Could you check a few things on this model? Use its own coordinates, in mm. A direction names the side the tool comes from. Give positions to 0.01 mm unless a question says otherwise; leave off trailing zeros. Order: outer loops, then holes, each group sorted by start corner. A loop starts at its lowest first (then second) coordinate and runs counter-clockwise, first axis right, second up. Notation, with made-up numbers: (-9.75, 3) -> (47.25, 3) arc R18 cw to (47.25, 23) -> close; hole circle Ø2 at (7.25, 51). An arc over 180 degrees is marked (long way). Use one line per item in the form item = value. Start each with the question number.
from build123d import *

# Parameters (mm, degrees)
SKETCH1_W                                           = 67.31
SKETCH1_H                                           = 88.9
EXTRUDE1_DEPTH                                      = 12.7
SKETCH2_R                                           = 18.1356
EXTRUDE2_DEPTH                                      = 13.7
SKETCH3_W                                           = 28.468633454
SKETCH3_H                                           = 1.016
EXTRUDE3_DEPTH                                      = 13.7
F_1_4_CLEARANCE_HOLE1_D                             = 6.7564
CSK_FOR_1_2_FLAT_HEAD_MACHINE_SCREW_100_D           = 13.49248
CSK_FOR_1_2_FLAT_HEAD_MACHINE_SCREW_100_CSINK_D     = 25.8318
CSK_FOR_1_2_FLAT_HEAD_MACHINE_SCREW_100_CSINK_ANGLE = 100
SKETCH10_W                                          = 15.24
SKETCH10_H                                          = 31.75
EXTRUDE4_DEPTH                                      = 13.7
FILLET1_R                                           = 2.54
FILLET1_OF_MIRROR2_R                                = 2.54


with BuildPart() as part:
    # Sketch1 → Extrude1 (new body)
    with BuildSketch(Plane.XY):
        Rectangle(SKETCH1_W, SKETCH1_H)
    extrude(amount=EXTRUDE1_DEPTH)

    # Sketch2 → Extrude2 (cut, through all)
    with BuildSketch(Plane.XY.offset(12.7)):
        with Locations((-9.525, 0)):
            Circle(SKETCH2_R)
    extrude(amount=-EXTRUDE2_DEPTH, mode=Mode.SUBTRACT)

    # Sketch3 → Extrude3 (cut, through all)
    with BuildSketch(Plane.XY.offset(12.7)):
        with Locations((21.1328, 0)):
            Rectangle(SKETCH3_W, SKETCH3_H)
    extrude(amount=-EXTRUDE3_DEPTH, mode=Mode.SUBTRACT)

    # 1/4 Clearance Hole1 (through all)
    with Locations(Plane(origin=(27.305, 44.45, 6.35), x_dir=(0, 0, 1), z_dir=(0, 1, 0))):
        with Locations((0, 0)):
            Hole(F_1_4_CLEARANCE_HOLE1_D / 2)

    # CSK for 1/2 Flat Head Machine Screw (100)1 (through all)
    with Locations(Plane(origin=(-20.955, 31.75, 12.7), x_dir=(1, 0, 0), z_dir=(0, 0, 1))):
        with Locations((0, 0)):
            csk_for_1_2_flat_head_machine_screw_100 = CounterSinkHole(CSK_FOR_1_2_FLAT_HEAD_MACHINE_SCREW_100_D / 2, CSK_FOR_1_2_FLAT_HEAD_MACHINE_SCREW_100_CSINK_D / 2, counter_sink_angle=CSK_FOR_1_2_FLAT_HEAD_MACHINE_SCREW_100_CSINK_ANGLE)

    # Mirror1: CSK for 1/2 Flat Head Machine Screw (100)1 across plane
    add(csk_for_1_2_flat_head_machine_screw_100.mirror(Plane.ZX), mode=Mode.SUBTRACT)

    # Sketch10 → Extrude4 (cut, through all)
    with BuildSketch(Plane.XY.offset(12.7)):
        with Locations((26.035, 28.575)):
            Rectangle(SKETCH10_W, SKETCH10_H)
    extrude4 = extrude(amount=-EXTRUDE4_DEPTH, mode=Mode.SUBTRACT)

    # Fillet1
    fillet1_edges = [part.edges().sort_by_distance(p)[0] for p in [
        (18.415, 12.7, 6.35),
    ]]
    fillet(fillet1_edges, radius=FILLET1_R)

    # Mirror2: Extrude4 across plane
    add(extrude4.mirror(Plane.ZX), mode=Mode.SUBTRACT)

    # Fillet1 of Mirror2
    fillet1_of_mirror2_edges = [part.edges().sort_by_distance(p)[0] for p in [
        (18.415, -12.7, 6.35),
    ]]
    fillet(fillet1_of_mirror2_edges, radius=FILLET1_OF_MIRROR2_R)


solid = part.part
(1) Imagine slicing it at D-D (x = -15.5). Give the number of separate pieces and of enclosed holes in the cut face, plus the area to 3 significant figures.
(2) I'm going to push flat-ended pins straight in: pin 1 Ø6.5 at (x, z) = (27.5, 6) entering from +Y; pin 2 Ø4 at (x, z) = (22, 7) entering from -Y; pin 3 Ø6.5 at (x, z) = (29, 5) entering from -Y. Where does each tip first touch, or does it pass through?
(3) Which directions (+Z, -Z, +X, -X, +Y, -Y) give clear straight access to the entire face, cutting with the end or side of a thin tool? Please do faces 4 (the cylindrical face through (-24.58, -37.44, 3.71)), 5 (the flat face through (30, 12.7, 4)), 6 (the flat face through (30, -12.7, 4)).
(4) Imagine slicing it at C-C (x = 25). Write out the boundary of the cut face in (y, z).
(5) We'd pull the mould along Z, two halves only. Please class faces 1 (the flat face through (7, -9, 12.7)), 2 (the flat face through (21, 0.508, 6)), 3 (the cylindrical face through (30.654, -6.689, 6.79)): pulls with the +Z half, pulls with the -Z half, needs draft (parallel to the pull), parting line crosses it, or undercut.
(6) Please list where these lines run through material, in increasing order: probe 1 along X at (y, z) = (31.75, 2) (3 decimals); probe 2 along Y at (x, z) = (-18.5, 6); probe 3 along X at (y, z) = (3.75, 6.35) (3 decimals).
(7) Imagine slicing it at A-A (z = 6.35). Write out the boundary of the cut face in (x, y) (3 decimals), plus the area to 3 significant figures.
(8) Imagine slicing it at B-B (y = -31.75). Write out the boundary of the cut face in (x, z) (3 decimals).
Calculated:
q1.separate_pieces = 4
q1.enclosed_holes = 0
q1.area = 407 mm2
q2.pin_1 = 12.7
q2.pin_2 = -12.89
q2.pin_3 = -12.7
q3.face_4 = +Z, -Z
q3.face_5 = +Z, -Z, +X, +Y
q3.face_6 = +Z, -Z, +X, -Y
q4.outline = (-12.7, 0) -> (-0.51, 0) -> (-0.51, 3.88) -> (-12.7, 3.88) -> close; (-12.7, 8.82) -> (-0.51, 8.82) -> (-0.51, 12.7) -> (-12.7, 12.7) -> close; (0.51, 0) -> (12.7, 0) -> (12.7, 3.88) -> (0.51, 3.88) -> close; (0.51, 8.82) -> (12.7, 8.82) -> (12.7, 12.7) -> (0.51, 12.7) -> close
q5.face_1 = pulls with the +Z half
q5.face_2 = needs draft
q5.face_3 = undercut
q6.probe_1 = -33.655 to -27.701, -14.209 to 18.415
q6.probe_2 = -44.45 to -38.03, -25.47 to -15.76, 15.76 to 25.47, 38.03 to 44.45
q6.probe_3 = -33.655 to -27.269, 8.219 to 23.927, 30.683 to 33.655
q7.outline = (-33.655, -44.45) -> (18.415, -44.45) -> (18.415, -15.24) arc R2.54 cw to (20.955, -12.7) -> (23.927, -12.7) -> (23.927, -0.508) -> (8.603, -0.508) arc R18.136 cw (long way) to (8.603, 0.508) -> (23.927, 0.508) -> (23.927, 12.7) -> (20.955, 12.7) arc R2.54 cw to (18.415, 15.24) -> (18.415, 44.45) -> (-33.655, 44.45) -> close; (30.683, -12.7) -> (33.655, -12.7) -> (33.655, -0.508) -> (30.683, -0.508) -> close; (30.683, 0.508) -> (33.655, 0.508) -> (33.655, 12.7) -> (30.683, 12.7) -> close; hole circle Ø13.492 at (-20.955, -31.75); hole circle Ø13.492 at (-20.955, 31.75)
q7.area = 3,510 mm2
q8.outline = (-33.655, 0) -> (-27.701, 0) -> (-27.701, 7.523) -> (-33.655, 12.519) -> close; (-14.209, 0) -> (18.415, 0) -> (18.415, 12.7) -> (-8.039, 12.7) -> (-14.209, 7.523) -> close
